Could you check a few things on this model? Use its own coordinates, in mm. A direction names the side the tool comes from. Coordinates: 2 decimals unless noted, no trailing zeros. Loops run counter-clockwise (first coordinate to the right, second up) from the corner with the lowest first, then second, coordinate; pieces in that order, holes last.
1) For faces 1 (the face through (-8.675, 57, 2)), 2 (the face through (0, 72.975, 2)), 3 (the face through (-11.561, 56.186, 1.61)), 4 (the face through (5.5, 71, 2)), which set-ups out of +Z, -Z, +X, -X, +Y, -Y let a thin tool reach every point of the face, with its end or its side?
2) Imagine slicing it at A-A on y = 65. Please give me the cut outline in (x, z) (3 decimals), plus the area to 3 significant figures.
3) If I drill on line 1 along Y through (x, z) = (0.5, 0.25); line 2 along X through (y, z) = (78, 1.95); line 3 along X through (y, z) = (66, 2.55) (3 decimals), over which ranges is the centre line in solid material (lowest first)?
4) Imagine slicing it at B-B on z = 0.7. Please give me the cut outline in (x, y) (1 decimal), plus the area to 3 significant figures.
5) Imagine slicing it at D-D on x = 7. Please give me the cut outline in (y, z) (3 decimals).
6) Will these pins go through, and if not, where does the flat tip stop? P1, Ø1.6, axis at y = 75, z = 1, coming from the -X side; P2, Ø1, axis at y = 72, z = 1, coming from the +X side; P3, Ø1, axis at y = 58, z = 2, coming from the +X side.
7) Thinking about a two-plate mould opening in X: for faces 5 (the face through (7, 59.562, 2)), 6 (the face through (11.62, 56.28, 1.61)), 7 (the face through (0, 79.562, 2)), 8 (the face through (-12.675, 61, 2)), which applies, released by +X, released by -X, zero draft, split by the parting line, or undercut?
8) Imagine slicing it at C-C on y = 49.5. Please give me the cut outline in (x, z) (3 decimals), plus the area to 3 significant figures.
```python
from build123d import *

# Parameters (mm, degrees)
BOSS_EXTRUDE1_DEPTH = 3.175
SKETCH2_W           = 3.175
SKETCH2_H           = 3.175
CUT_EXTRUDE1_DEPTH  = 81.096853282
SKETCH3_W           = 3.175
SKETCH3_H           = 15
BOSS_EXTRUDE2_DEPTH = 4
FILLET1_R           = 7


with BuildPart() as part:
    # Sketch1 → Boss-Extrude1 (new body)
    with BuildSketch(Plane.XY):
        Polygon((3, 45.562363311), (-3, 45.562363311), (-5.5, 45.562363311), (-5.5, 59.562363311), (-8.675, 59.562363311), (-8.675, 62.737363311), (-5.5, 62.737363311), (-5.5, 79.562363311), (5.5, 79.562363311), (5.5, 62.737363311), (8.675, 62.737363311), (8.675, 59.562363311), (5.5, 59.562363311), (5.5, 45.562363311), align=None)
    extrude(amount=BOSS_EXTRUDE1_DEPTH)

    # Sketch2 → Cut-Extrude1 (cut, through all)
    with BuildSketch(Plane(origin=(0, 0, 0), x_dir=(-1, 0, 0), z_dir=(0, 0, -1))):
        with Locations((0, 74.562363311)):
            Rectangle(SKETCH2_W, SKETCH2_H)
    extrude(amount=-CUT_EXTRUDE1_DEPTH, mode=Mode.SUBTRACT)

    # Sketch3 → Boss-Extrude2 (add)
    with BuildSketch(Plane.ZY.offset(8.675)):
        with Locations((1.5875, 61.149863311)):
            Rectangle(SKETCH3_W, SKETCH3_H)
    boss_extrude2 = extrude(amount=BOSS_EXTRUDE2_DEPTH)

    # Mirror2: Boss-Extrude2 across plane
    add(boss_extrude2.mirror(Plane(origin=(0, 0, 0), x_dir=(0, 0, 1), z_dir=(1, 0, 0))))

    # Fillet1
    # the kernel refuses this fillet: 7 mm, written as the material it takes off along each edge
    with BuildSketch(Plane(origin=(-12.675, 68.649863311, -15.811388301), x_dir=(1, 0, 0), z_dir=(0, 0, 1))) as fillet1_piece_1:
        with BuildLine():
            CenterArc((7, -6.32455532), FILLET1_R, 115.376933525, 64.623066475)
            Line((0, -6.32455532), (-0.14, -6.32455532))
            Line((-0.14, -6.32455532), (-0.14, 0))
            Line((-0.14, 0), (0, 0.14))
            ThreePointArc((0, 0.14), (2, 0.14), (3.94, 0.126491106))
            Line((3.94, 0.126491106), (4, 0))
        make_face()
    extrude(amount=34.797776602, mode=Mode.SUBTRACT)
    with BuildSketch(Plane(origin=(-12.675, 53.649863311, 18.986388301), x_dir=(0, 1, 0), z_dir=(0, 0, -1))) as fillet1_piece_2:
        with BuildLine():
            CenterArc((6.32455532, 7), FILLET1_R, 205.376933525, 64.623066475)
            Line((0, 4), (-0.126491106, 3.94))
            ThreePointArc((-0.126491106, 3.94), (-0.14, 2), (-0.14, 0))
            Line((-0.14, 0), (0, -0.14))
            Line((0, -0.14), (6.32455532, -0.14))
            Line((6.32455532, -0.14), (6.32455532, 0))
        make_face()
    extrude(amount=34.797776602, mode=Mode.SUBTRACT)
    with BuildSketch(Plane(origin=(12.675, 68.649863311, -15.811388301), x_dir=(0, -1, 0), z_dir=(0, 0, 1))) as fillet1_piece_3:
        with BuildLine():
            CenterArc((6.32455532, -7), FILLET1_R, 90, 64.623066475)
            Line((0, -4), (-0.126491106, -3.94))
            ThreePointArc((-0.126491106, -3.94), (-0.14, -2), (-0.14, 0))
            Line((-0.14, 0), (0, 0.14))
            Line((0, 0.14), (6.32455532, 0.14))
            Line((6.32455532, 0.14), (6.32455532, 0))
        make_face()
    extrude(amount=34.797776602, mode=Mode.SUBTRACT)
    with BuildSketch(Plane(origin=(12.675, 53.649863311, 18.986388301), x_dir=(-1, 0, 0), z_dir=(0, 0, -1))) as fillet1_piece_4:
        with BuildLine():
            CenterArc((7, 6.32455532), FILLET1_R, 180, 64.623066475)
            Line((0, 6.32455532), (-0.14, 6.32455532))
            Line((-0.14, 6.32455532), (-0.14, 0))
            Line((-0.14, 0), (0, -0.14))
            ThreePointArc((0, -0.14), (2, -0.14), (3.94, -0.126491106))
            Line((3.94, -0.126491106), (4, 0))
        make_face()
    extrude(amount=34.797776602, mode=Mode.SUBTRACT)


solid = part.part
```
Filled in:
1. face 1: +Z, -Z, -Y
1. face 2: +Z, -Z
1. face 3: +Z, -Z, -X, -Y
1. face 4: +Z, -Z, +Y
2. outline: (-12.144, 0) - (-8.675, 0) - (-8.675, 3.175) - (-12.144, 3.175) - close; (-5.5, 0) - (5.5, 0) - (5.5, 3.175) - (-5.5, 3.175) - close; (8.675, 0) - (12.144, 0) - (12.144, 3.175) - (8.675, 3.175) - close
2. area: 57.0 mm2
3. line 1: y = 45.56 to 72.97, 76.15 to 79.56
3. line 2: x = -5.5 to 5.5
3. line 3: x = -11.633 to -8.675, -5.5 to 5.5, 8.675 to 11.633
4. outline: (-12.7, 60) arc R7 ccw to (-8.7, 53.6) - (-8.7, 59.6) - (-5.5, 59.6) - (-5.5, 45.6) - (5.5, 45.6) - (5.5, 59.6) - (8.7, 59.6) - (8.7, 53.6) arc R7 ccw to (12.7, 60) - (12.7, 62.3) arc R7 ccw to (8.7, 68.6) - (8.7, 62.7) - (5.5, 62.7) - (5.5, 79.6) - (-5.5, 79.6) - (-5.5, 62.7) - (-8.7, 62.7) - (-8.7, 68.6) arc R7 ccw to (-12.7, 62.3) - close; hole (-1.6, 73) - (1.6, 73) - (1.6, 76.1) - (-1.6, 76.1) - close
4. area: 475 mm2
5. outline: (59.562, 0) - (62.737, 0) - (62.737, 3.175) - (59.562, 3.175) - close
6. P1: stops at x = -5.5
6. P2: stops at x = 5.5
6. P3: stops at x = 12.52
7. face 5: undercut
7. face 6: released by +X
7. face 7: zero draft
7. face 8: released by -X
8. outline: (-5.5, 0) - (5.5, 0) - (5.5, 3.175) - (-5.5, 3.175) - close
8. area: 34.9 mm2
